from build123d import *

# Parameters (mm, degrees)
F0_W     = 9
F0_H     = 3
F2_SIZE2 = 2
F2_SIZE  = 2


with BuildPart() as f1:
    # F0 (on Front) → F1 (revolve)
    with BuildSketch(Plane.XZ):
        Polygon((0, 47.565076), (0, 10.565076), (9, 10.565076), (11, 10.565076), (11, 47.565076), align=None)
        with Locations((4.5, 9.065076)):
            Rectangle(F0_W, F0_H)
        Polygon((0, 7.565076), (0, -7.434924), (14, -7.434924), (14, 7.565076), (9, 7.565076), align=None)
        Polygon((0, -7.434924), (0, -32.434924), (21, -32.434924), (21, -7.434924), (14, -7.434924), align=None)
    revolve(axis=Axis((0, 0, 7.565076), (0, 0, -1)))

    # F2
    f2_edges = [f1.edges().sort_by_distance(p)[0] for p in [
        (-11, 0, 47.565076),
        (-21, 0, -32.434924),
    ]]
    chamfer(f2_edges, length=F2_SIZE, length2=F2_SIZE2)


solid = f1.part
Could you check a few things on this model? Use its own coordinates, in mm. A direction names the side the tool comes from. Round coordinates to 2 decimals unless told otherwise and drop trailing zeros. Order: outer loops, then holes, each group sorted by start corner. A loop starts at its lowest first (then second) coordinate and runs counter-clockwise, first axis right, second up.
(1) Please list where these lines run through material, in increasing order: line 1 along Z through (x, y) = (9.5, 14); line 2 along Z through (x, y) = (2, 13.5); line 3 along Y through (x, z) = (0, 42).
Response values:
line 1: z = -32.43 to -7.43
line 2: z = -32.43 to 7.57
line 3: y = -11 to 11
(2) I'm going to push flat-ended pins straight in: pin 1 (10 mm diameter, centred on y = 0.5, z = 28.5, fed in from +X); pin 2 (3 mm diameter, centred on y = -15, z = -7.5, fed in from +X); pin 3 (1.5 mm diameter, centred on x = -10.5, z = -4, fed in from -Y). Where does each tip first touch, or does it pass through?
Response values:
pin 1: stops at x = 11
pin 2: stops at x = 16.09
pin 3: stops at y = -10.05
(3) If we mould it in two halves opening along Z, with no side actions, what happens to faces 1 (the cylindrical face through (-1.172, -8.923, 9.086)), 2 (the cylindrical face through (12.932, 5.362, 0.17)), 3 (the flat face through (0, 0, -32.435))? For each: released by +Z, released by -Z, zero draft, split by the parting line, or undercut.
Response values:
face 1: undercut
face 2: zero draft
face 3: released by -Z
(4) Imagine slicing it at A-A (y = 0). Write out the boundary of the cut face in (x, z), plus the area to 3 significant figures.
Response values:
outline: (-21, -30.43) - (-19, -32.43) - (19, -32.43) - (21, -30.43) - (21, -7.43) - (14, -7.43) - (14, 7.57) - (9, 7.57) - (9, 10.57) - (11, 10.57) - (11, 45.57) - (9, 47.57) - (-9, 47.57) - (-11, 45.57) - (-11, 10.57) - (-9, 10.57) - (-9, 7.57) - (-14, 7.57) - (-14, -7.43) - (-21, -7.43) - close
area: 2,330 mm2
(5) Imagine slicing it at C-C (z = -16). Write out the boundary of the cut face in (x, y), plus the area to 3 significant figures.
Response values:
outline: circle Ø42 at (0, 0)
area: 1,390 mm2
(6) Imagine slicing it at D-D (z = 38). Write out the boundary of the cut face in (x, y).
Response values:
outline: circle Ø22 at (0, 0)
(7) Which directions (+Z, -Z, +X, -X, +Y, -Y) give clear straight access to the entire face, cutting with the end or side of a thin tool? Please do faces 4 (the flat face through (9, 3, 7.565)), 5 (the conical face through (-4.15, 18.67, -32.31)), 6 (the flat face through (4, 14, -7.435)).
Response values:
face 4: none
face 5: -Z
face 6: +Z
